```python
from build123d import *

# Parameters (mm, degrees)
F1_DEPTH = 25
F3_DEPTH = 100
F4_DEPTH = 100


with BuildPart() as f1:
    # F0 (on Top) → F1 (new body)
    with BuildSketch(Plane.XY):
        Polygon((58, 0), (0, 0), (0, -93.7), (40.9, -93.7), (40.9, -87.8), (43.5, -85.2), (49.7, -85.2), (49.7, -83.4), (46.3, -83.4), (46.3, -50), (53.3, -43), (58, -43), align=None)
    extrude(amount=F1_DEPTH)

    # F3 (add): a face of the model
    f3_faces = [f1.faces().sort_by_distance(p)[0] for p in [
        (26.1504271655, -43.8715742384, 25),
    ]]
    extrude(f3_faces, amount=F3_DEPTH)

    # F2 (on face) → F4 (join)
    with BuildSketch(Plane(origin=(0, 0, 0), x_dir=(0, -1, 0), z_dir=(-1, 0, 0))):
        Polygon((0, 24.2), (0, 0), (93.7, 0), (93.7, 7.1), (87.8, 7.1), (85.2, 9.7), (85.2, 19.4), (83.4, 19.4), (83.4, 12.4), (50, 12.4), (43, 19.4), (43, 24.2), align=None)
    extrude(amount=-F4_DEPTH)


solid = f1.part
```
Could you check a few things on this model? Use its own coordinates, in mm. A direction names the side the tool comes from. Coordinates: 2 decimals unless noted, no trailing zeros. Write each loop counter-clockwise with the first axis right and the second up, starting at its lowest first coordinate (ties: lowest second). Pieces come first, ordered by that corner, then holes. Notation, with made-up numbers: M 83,77.5 L 130,77.5 A31 ccw 130,110.5 Z; hole C 26.25,43.5 d5. An arc over 180 degrees is marked long. Answer as CSV lines item,"result". Start each with the question number.
1) For faces 1 (the flat face through (79, -22, 24.2)), 2 (the flat face through (72.8, -46.5, 15.9)), 3 (the flat face through (49, -46, 0)), 4 (the flat face through (29, -46, 125)), 5 (the flat face through (40.9, -91, 65)), which set-ups out of +Z, -Z, +X, -X, +Y, -Y let a thin tool reach every point of the face, with its end or its side?
2) For P1, Ø16.5, axis at y = -72, z = 84, coming from the +X side; P2, Ø1.8, axis at y = -92, z = 38.5, coming from the +X side; P3, Ø6.5, axis at x = 60, y = -92, coming from the +Z side, each with a flat end and sliding along its axis, tell me the tip position at first contact or that it passes through.
3) I want a section at A-A, the plane x = 65. Please give me the cut outline in (y, z), and give its area (3 significant figures).
4) I want a section at D-D, the plane y = -62.5. Please give me the cut outline in (x, z).
5) Please list where these lines run through material, in increasing order: line 1 (Z direction, x = 57.5, y = -73.5); line 2 (X direction, y = -67, z = 62); line 3 (X direction, y = -12, z = 96). Write a range as from..to.
6) I want a section at B-B, the plane z = 16. Please give me the cut outline in (x, y), and give its area (3 significant figures).
7) We'd pull the mould along Y, two halves only. Please class faces 6 (the flat face through (0, -46, 62)), 7 (the flat face through (40, 0, 48)), 8 (the flat face through (49, -83.4, 44)): +Y half, -Y half, draft (parallel to the pull), parting line (faces both ways), or undercut.
8) I want a section at C-C, the plane y = -17. Please give me the cut outline in (x, z), and give its area (3 significant figures).
Data:
1,face 1,"+Z, +X, +Y, -Y"
1,face 2,"+Z, +X"
1,face 3,"-Z, +X, -X, +Y, -Y"
1,face 4,"+Z, +X, -X, +Y, -Y"
1,face 5,"+Z, +X, -Y"
2,P1,"stops at x = 46.3"
2,P2,"stops at x = 40.9"
2,P3,"stops at z = 7.1"
3,outline,"M -93.7,0 L 0,0 L 0,24.2 L -43,24.2 L -43,19.4 L -50,12.4 L -83.4,12.4 L -83.4,19.4 L -85.2,19.4 L -85.2,9.7 L -87.8,7.1 L -93.7,7.1 Z"
3,area,"1,660 mm^2"
4,outline,"M 0,0 L 100,0 L 100,12.4 L 46.3,12.4 L 46.3,125 L 0,125 Z"
5,line 1,"z = 0..12.4"
5,line 2,"x = 0..46.3"
5,line 3,"x = 0..58"
6,outline,"M 0,-93.7 L 40.9,-93.7 L 40.9,-87.8 L 43.5,-85.2 L 100,-85.2 L 100,-83.4 L 46.3,-83.4 L 46.3,-50 L 49.9,-46.4 L 100,-46.4 L 100,0 L 0,0 Z"
6,area,"6,890 mm^2"
7,face 6,"draft"
7,face 7,"+Y half"
7,face 8,"undercut"
8,outline,"M 0,0 L 100,0 L 100,24.2 L 58,24.2 L 58,125 L 0,125 Z"
8,area,"8,270 mm^2"
